from build123d import *

# Parameters (mm, degrees)
SKETCH1_W            = 7.62
SKETCH1_H            = 10.6
BOSS_EXTRUDE1_DEPTH  = 5.15
SKETCH3_R            = 0.29
BOSS_EXTRUDE2_DEPTH  = 2.54
LPATTERN1_COUNT      = 3
LPATTERN1_PITCH      = 2.54
LPATTERN1_COUNT_DIR2 = 2
LPATTERN1_PITCH_DIR2 = 7.62
CUT_EXTRUDE1_DEPTH   = 11.614937588


with BuildPart() as part:
    # Sketch1 → Boss-Extrude1 (new body)
    with BuildSketch(Plane(origin=(0, 0, 0), x_dir=(1, 0, 0), z_dir=(0, 1, 0))):
        Rectangle(SKETCH1_W, SKETCH1_H)
    extrude(amount=BOSS_EXTRUDE1_DEPTH)

    # Sketch3 → Boss-Extrude2 (add)
    with BuildSketch(Plane.XZ):
        with Locations(Location((2.54, -3.81, 0), (0, 0, 270))):
            Circle(SKETCH3_R)
    boss_extrude2 = extrude(amount=BOSS_EXTRUDE2_DEPTH)

    # LPattern1: Boss-Extrude2 3 × 2
    with Locations(*[(-i * LPATTERN1_PITCH, 0, j * LPATTERN1_PITCH_DIR2) for i in range(LPATTERN1_COUNT) for j in range(LPATTERN1_COUNT_DIR2) if (i, j) != (0, 0)]):
        add(boss_extrude2)

    # Sketch4 → Cut-Extrude1 (cut, through all)
    with BuildSketch(Plane.ZY.offset(3.81)):
        Polygon((-5.08, 5.15), (-4.7625, 4.15), (4.7625, 4.15), (5.08, 5.15), align=None)
    extrude(amount=-CUT_EXTRUDE1_DEPTH, mode=Mode.SUBTRACT)


solid = part.part
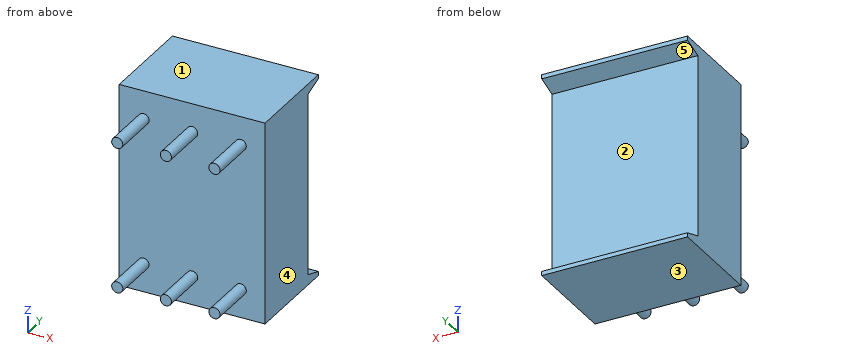
Verification items for the finished model (mm, model axes). Face numbers are marked on the shaded views. A direction names the side the tool comes from. Give positions to 0.01 mm unless a question says otherwise; leave off trailing zeros. Loops run counter-clockwise (first coordinate to the right, second up) from the corner with the lowest first, then second, coordinate; pieces in that order, holes last.
1) Depth check by flat-ended pin: pin 1 Ø4 at (y, z) = (-0.5, 4) entering from -X; pin 2 Ø1 at (x, z) = (0.5, 2) entering from -Y. Enter the tip coordinate at first touch or a pass-through.
2) Sectioned sample at D-D, the plane z = -3.25. Enter the section's corners in (x, y).
3) Sectioned sample at B-B, the plane z = 3.81. Enter the section's corners in (x, y), then the cut area to 3 significant figures.
4) Set-up check for the marked faces 4 and 5: record each of +Z, -Z, +X, -X, +Y, -Y from which the full face is reachable in a straight line by a thin tool's end or side.
5) Sectioned sample at A-A, the plane x = -1.5. Enter the section's corners in (y, z), then the cut area to 3 significant figures.
6) Draft check along Z on the marked faces 1, 2 and 3. Enter one of: pulls with the +Z half, pulls with the -Z half, needs draft (parallel to the pull), parting line crosses it, or undercut.
7) Thickness scan on line 1 along Z through (x, y) = (-2.5, -0.75); line 2 along Y through (x, z) = (-1.5, 3.75); line 3 along X through (y, z) = (-0.25, 4). Record the ranges inside material, lowest first.
8) Sectioned sample at C-C, the plane x = 2.54. Enter the section's corners in (y, z).
Answers:
1. pin 1: stops at x = -3.81
1. pin 2: stops at y = 0
2. outline: (-3.81, 0) - (3.81, 0) - (3.81, 4.15) - (-3.81, 4.15) - close
3. outline: (-3.81, 0) - (-2.83, 0) - (-2.83, -2.54) - (-2.25, -2.54) - (-2.25, 0) - (-0.29, 0) - (-0.29, -2.54) - (0.29, -2.54) - (0.29, 0) - (2.25, 0) - (2.25, -2.54) - (2.83, -2.54) - (2.83, 0) - (3.81, 0) - (3.81, 4.15) - (-3.81, 4.15) - close
3. area: 36.0 mm2
4. face 4: +Z, -Z, +X, +Y, -Y
4. face 5: +X, -X, +Y
5. outline: (0, -5.3) - (5.15, -5.3) - (5.15, -5.08) - (4.15, -4.76) - (4.15, 4.76) - (5.15, 5.08) - (5.15, 5.3) - (0, 5.3) - close
5. area: 44.7 mm2
6. face 1: pulls with the +Z half
6. face 2: undercut
6. face 3: pulls with the -Z half
7. line 1: z = -4.1 to -3.52, 3.52 to 4.1
7. line 2: y = 0 to 4.15
7. line 3: x = -2.76 to -2.32, -0.22 to 0.22, 2.32 to 2.76
8. outline: (-2.54, -4.1) - (0, -4.1) - (0, -5.3) - (5.15, -5.3) - (5.15, -5.08) - (4.15, -4.76) - (4.15, 4.76) - (5.15, 5.08) - (5.15, 5.3) - (0, 5.3) - (0, 4.1) - (-2.54, 4.1) - (-2.54, 3.52) - (0, 3.52) - (0, -3.52) - (-2.54, -3.52) - close
